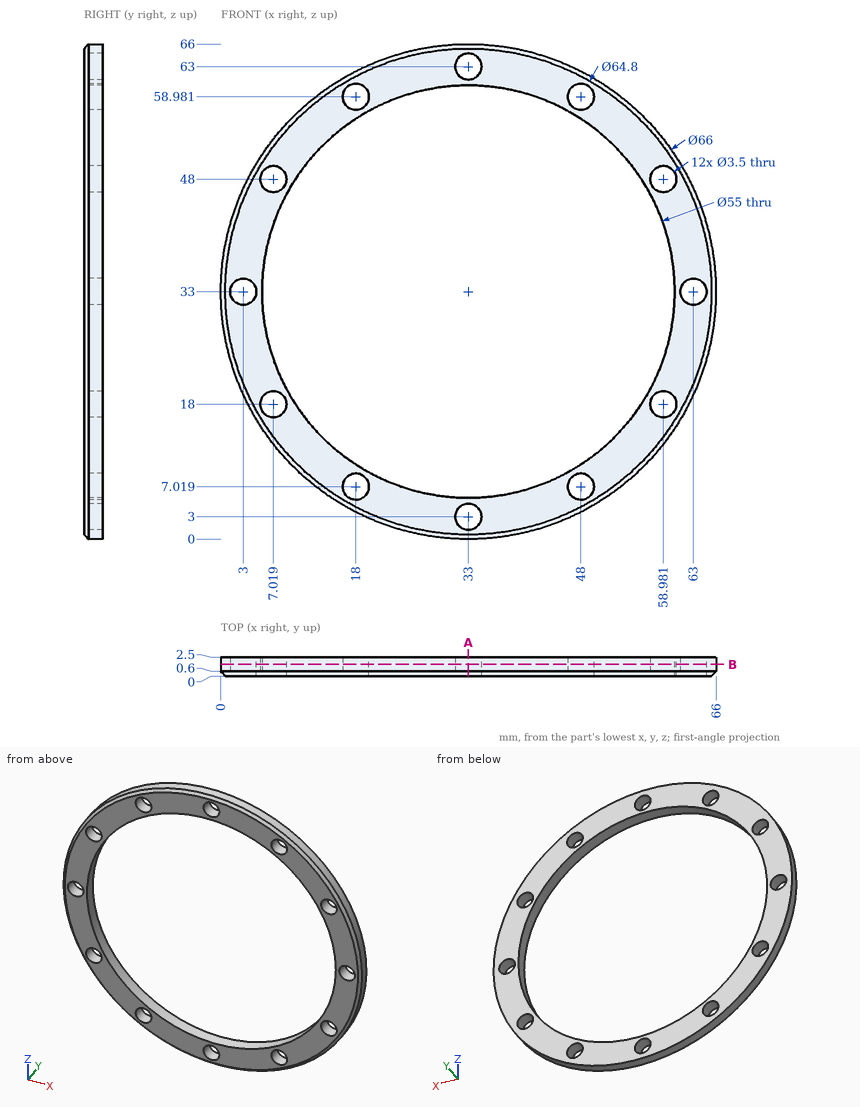
Design review of the part shown in the three views and the two pictorial views. Dimensions are in mm from the part's minimum x, y and z. Round coordinates to 2 decimals unless told otherwise and drop trailing zeros. Write each loop counter-clockwise with the first axis right and the second up, starting at its lowest first coordinate (ties: lowest second). Pieces come first, ordered by that corner, then holes. Notation, with made-up numbers: (62, 13.5) -> (89, 13.5) arc R12 cw to (89, 21.5) -> close; hole circle Ø10 at (89, 31.25). An arc over 180 degrees is marked (long way). One line per question, with ' | ' between items. Start each with the question number.
1) Add section B-B (y = 1.55). Count the separate pieces of the cut face and the enclosed holes in it, and give its area (3 significant figures).
2) Wall thickness on line 1 along X through (y, z) = (1, 33); line 2 along Z through (x, y) = (18, 1.75); line 3 along X through (y, z) = (2.1, 51.5): over which ranges is each line inside the solid? List them lowest first.
3) For pin 1 Ø1.5 at (y, z) = (1, 27) entering from -X, flat-tipped, find the tip position at first contact; note if it passes through.
4) Add section A-A (x = 33). Write out the cut boundary in (y, z).
Reported:
1) separate pieces: 1 | enclosed holes: 13 | area: 930 mm²
2) line 1: x = 0 to 1.25, 4.75 to 5.5, 60.5 to 61.25, 64.75 to 66 | line 2: z = 3.61 to 5.27, 8.77 to 9.95, 56.05 to 57.23, 60.73 to 62.39 | line 3: x = 5.67 to 12.65, 53.35 to 60.33
3) pin 1: stops at x = 0.42
4) outline: (0, 0.6) -> (0.6, 0) -> (2.5, 0) -> (2.5, 1.25) -> (0, 1.25) -> close; (0, 4.75) -> (2.5, 4.75) -> (2.5, 5.5) -> (0, 5.5) -> close; (0, 60.5) -> (2.5, 60.5) -> (2.5, 61.25) -> (0, 61.25) -> close; (0, 64.75) -> (2.5, 64.75) -> (2.5, 66) -> (0.6, 66) -> (0, 65.4) -> close
